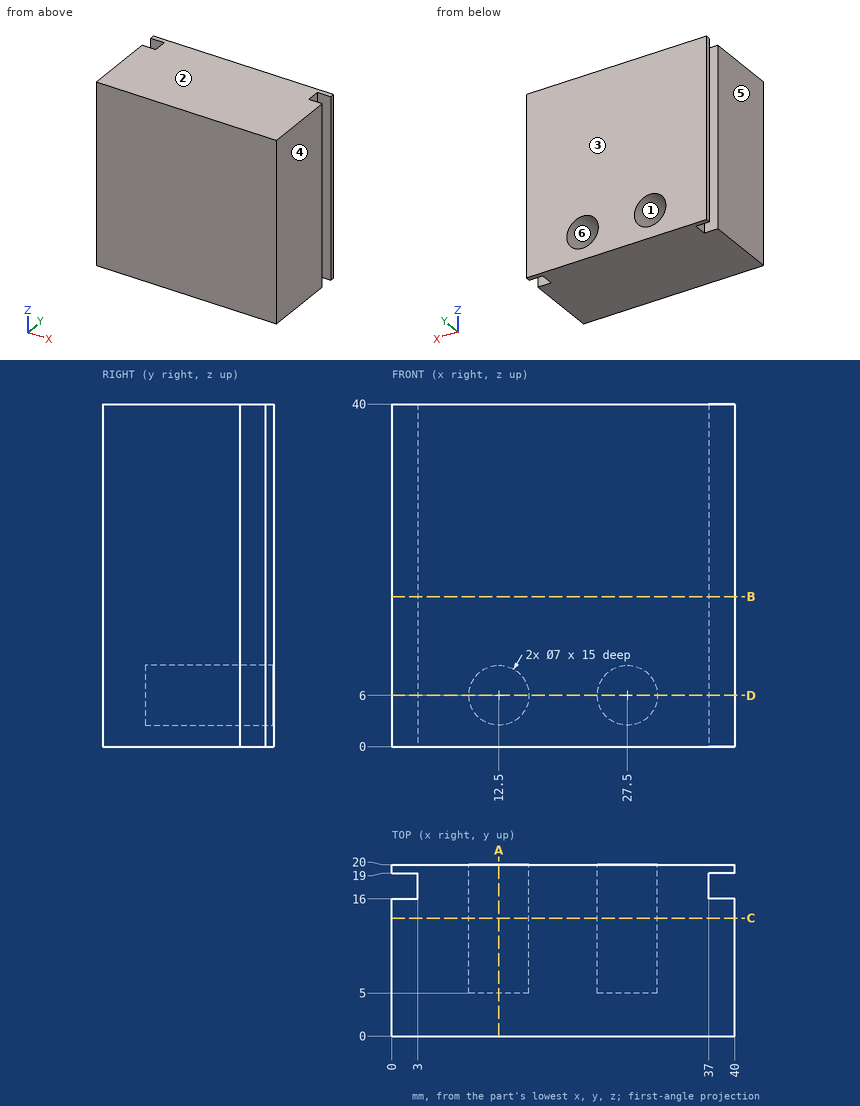
Could you check a few things on this drawing? It's one solid part, dimensions in mm from its lowest x, y, z. A direction names the side the tool comes from. Give positions to 0.01 mm unless a question says otherwise; leave off trailing zeros. Order: outer loops, then holes, each group sorted by start corner. A loop starts at its lowest first (then second) coordinate and runs counter-clockwise, first axis right, second up. Notation, with made-up numbers: (-35.5, -13.5) -> (12.5, -13.5) arc R18 cw to (12.5, 4.5) -> close; hole circle Ø5 at (-35, 48). An arc over 180 degrees is marked (long way). Answer in a Markdown table with one row per item. Add a question column.
Item 1: Imagine slicing it at B-B (z = 17.5). List the corners of the cut face in (x, y) for me.
Item 2: For the marked faces 1 and 2, which set-ups out of +Z, -Z, +X, -X, +Y, -Y let a thin tool reach every point of the face, with its end or its side?
Item 3: Please list where these lines run through material, in increasing order: probe 1 along X at (y, z) = (12.75, 6); probe 2 along X at (y, z) = (17.25, 6); probe 3 along Y at (x, z) = (2.5, 10).
Item 4: Imagine slicing it at C-C (y = 13.75). List the corners of the cut face in (x, z) for me.
Item 5: We'd pull the mould along X, two halves only. Please class the marked faces 3, 4, 5 and 6: pulls with the +X half, pulls with the -X half, needs draft (parallel to the pull), parting line crosses it, or undercut.
Item 6: I'm going to push a flat-ended pin straight in: P1, Ø3.5, axis at x = 12, z = 6.5, coming from the +Y side. Where does the tip first touch, or does it pass through?
Item 7: Imagine slicing it at D-D (z = 6). List the corners of the cut face in (x, y) for me.
Item 8: Imagine slicing it at A-A (x = 12.5). List the corners of the cut face in (y, z) for me.
Result:
| question | item | result |
|---|---|---|
| 1 | outline | (0, 0) -> (40, 0) -> (40, 16) -> (37, 16) -> (37, 19) -> (40, 19) -> (40, 20) -> (0, 20) -> (0, 19) -> (3, 19) -> (3, 16) -> (0, 16) -> close |
| 2 | face 1 | +Y |
| 2 | face 2 | +Z, +X, -X, +Y, -Y |
| 3 | probe 1 | 0 to 9, 16 to 24, 31 to 40 |
| 3 | probe 2 | 3 to 9, 16 to 24, 31 to 37 |
| 3 | probe 3 | 0 to 16, 19 to 20 |
| 4 | outline | (0, 0) -> (40, 0) -> (40, 40) -> (0, 40) -> close; hole circle Ø7 at (12.5, 6); hole circle Ø7 at (27.5, 6) |
| 5 | face 3 | needs draft |
| 5 | face 4 | pulls with the +X half |
| 5 | face 5 | pulls with the -X half |
| 5 | face 6 | undercut |
| 6 | P1 | y = 5 |
| 7 | outline | (0, 0) -> (40, 0) -> (40, 16) -> (37, 16) -> (37, 19) -> (40, 19) -> (40, 20) -> (31, 20) -> (31, 5) -> (24, 5) -> (24, 20) -> (16, 20) -> (16, 5) -> (9, 5) -> (9, 20) -> (0, 20) -> (0, 19) -> (3, 19) -> (3, 16) -> (0, 16) -> close |
| 8 | outline | (0, 0) -> (20, 0) -> (20, 2.5) -> (5, 2.5) -> (5, 9.5) -> (20, 9.5) -> (20, 40) -> (0, 40) -> close |
